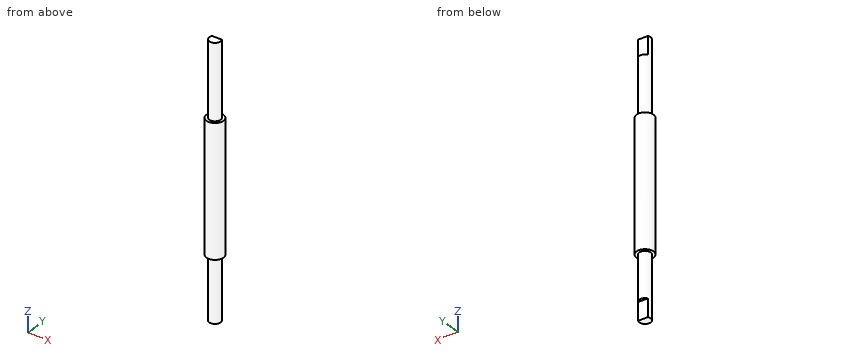
from build123d import *

# Parameters (mm, degrees)
SKETCH1_R           = 6.35
BOSS_EXTRUDE1_DEPTH = 300
BOSS_EXTRUDE2_START = -70.2975
SKETCH2_R           = 9.525
BOSS_EXTRUDE2_DEPTH = 146
CUT_EXTRUDE4_DEPTH  = 20
CUT_EXTRUDE5_START  = 280
CUT_EXTRUDE5_DEPTH  = 20


with BuildPart() as part:
    # Sketch1 → Boss-Extrude1 (new body)
    with BuildSketch(Plane.XY):
        Circle(SKETCH1_R)
    extrude(amount=BOSS_EXTRUDE1_DEPTH)

    # Sketch2 → Boss-Extrude2 (add)
    with BuildSketch(Plane(origin=(0, 0, 0), x_dir=(-1, 0, 0), z_dir=(0, 0, -1)).offset(BOSS_EXTRUDE2_START)):
        Circle(SKETCH2_R)
    extrude(amount=-BOSS_EXTRUDE2_DEPTH)

    # Sketch7 → Cut-Extrude4 (cut)
    with BuildSketch(Plane.XY):
        with BuildLine():
            Line((-5.499261314, 3.175), (5.499261314, 3.175))
            ThreePointArc((5.499261314, 3.175), (0, 6.35), (-5.499261314, 3.175))
        make_face()
    extrude(amount=CUT_EXTRUDE4_DEPTH, mode=Mode.SUBTRACT)

    # Sketch7<3> → Cut-Extrude5 (cut)
    with BuildSketch(Plane.XY.offset(CUT_EXTRUDE5_START)):
        with BuildLine():
            Line((-5.499261314, 3.175), (5.499261314, 3.175))
            ThreePointArc((5.499261314, 3.175), (0, 6.35), (-5.499261314, 3.175))
        make_face()
    extrude(amount=CUT_EXTRUDE5_DEPTH, mode=Mode.SUBTRACT)


solid = part.part
Work out the finished part from the listing and answer in its coordinate system (mm). Round coordinates to 2 decimals unless told otherwise and drop trailing zeros. Order: outer loops, then holes, each group sorted by start corner. A loop starts at its lowest first (then second) coordinate and runs counter-clockwise, first axis right, second up. Notation, with made-up numbers: M 23,-38 L 82,-38 A29 cw 82,-7 Z; hole C 70,83 d11. An arc over 180 degrees is marked long. One line per item, written item: value.
Q1. Flat-ended cylindrical pins translate along their axes: pin 1 (1.6 mm diameter, centred on x = 2, y = 5, fed in from +Z); pin 2 (1.5 mm diameter, centred on x = 7.5, z = 164, fed in from +Y); pin 3 (1.5 mm diameter, centred on y = 2.5, z = 93.5, fed in from +X). Find the tip coordinate at first contact, or state that the pin passes through.
Derived:
pin 1: z = 280
pin 2: y = 6.72
pin 3: x = 9.36
Q2. Find section C-C on z = 186.5. Write down the section's boundary in (x, y) (3 decimals), then the cut area to 3 significant figures.
Derived:
outline: C 0,0 d19.05
area: 285 mm²
Q3. Find section D-D on z = 228. Write down the section's boundary in (x, y).
Derived:
outline: C 0,0 d12.7
Q4. Straight lines are drawn through the part: line 1 (Z direction, x = 5.75, y = 7.25); line 2 (Y direction, x = 1.25, z = 104.5); line 3 (X direction, y = 6.5, z = 100.5). For each, find the intervals that lie inside material, in ascending order.
Derived:
line 1: 70.3 to 216.3
line 2: -9.44 to 9.44
line 3: -6.96 to 6.96
